```python
from build123d import *

# Parameters (mm, degrees)
SKETCH_1_R          = 4
EXTRUDE_1_DEPTH     = 26
SKETCH_2_R          = 4
EXTRUDE_2_DEPTH     = 36
SKETCH_3_R          = 1.5
CUT_EXTRUDE_1_DEPTH = 37.441734317
CHAMFER_1_SIZE      = 0.2


with BuildPart() as part:
    # ｽｹｯﾁ1 → ﾎﾞｽ - 押し出し1 (new, symmetric)
    with BuildSketch(Plane.XY):
        with Locations(Location((0, 0, 0), (0, 0, 180))):
            Circle(SKETCH_1_R)
    extrude(amount=EXTRUDE_1_DEPTH, both=True)

    # ｽｹｯﾁ2 → ﾎﾞｽ - 押し出し2 (add, symmetric)
    with BuildSketch(Plane.XY):
        with Locations(Location((0, 0, 0), (0, 0, 180))):
            Circle(SKETCH_2_R)
    extrude(amount=EXTRUDE_2_DEPTH, both=True)

    # ｽｹｯﾁ3 → ｶｯﾄ - 押し出し1 (cut, symmetric)
    with BuildSketch(Plane(origin=(0, 0, 0), x_dir=(1, 0, 0), z_dir=(0, 1, 0))):
        with Locations(Location((0, 30, 0), (0, 0, 270))):
            Circle(SKETCH_3_R)
    cut_extrude_1 = extrude(amount=CUT_EXTRUDE_1_DEPTH, both=True, mode=Mode.SUBTRACT)

    # ﾐﾗｰ1: ｶｯﾄ - 押し出し1 across plane
    add(cut_extrude_1.mirror(Plane.XY), mode=Mode.SUBTRACT)

    # 面取り1
    chamfer_1_edges = [part.edges().sort_by_distance(p)[0] for p in [
        (4, 0, -36),
        (4, 0, 36),
    ]]
    chamfer(chamfer_1_edges, length=CHAMFER_1_SIZE)


solid = part.part
```
Verification items for the finished model (mm, model axes). Give positions to 0.01 mm unless a question says otherwise; leave off trailing zeros. Loops run counter-clockwise (first coordinate to the right, second up) from the corner with the lowest first, then second, coordinate; pieces in that order, holes last. Notation, with made-up numbers: M 73,36 L 117,36 A15 ccw 117,64 Z; hole C 37.5,64 d4. An arc over 180 degrees is marked long. One line per question, with ' | ' between items.
Item 1: Section check A-A, the plane y = 0. Record the cut outline in (x, z), plus the area to 3 significant figures.
Completed:
outline: M -4,-35.8 L -3.8,-36 L 3.8,-36 L 4,-35.8 L 4,35.8 L 3.8,36 L -3.8,36 L -4,35.8 Z; hole C 0,-30 d3; hole C 0,30 d3 | area: 562 mm^2
Item 2: Draft check along X on faces 1 (the face through (0.867, 3.905, 0.501)), 2 (the face through (0, 0, -36)), 3 (the face through (0.07, 0.06, -31.5)). Enter one of: +X half, -X half, draft (parallel to the pull), parting line (faces both ways), or undercut.
Completed:
face 1: parting line | face 2: draft | face 3: undercut
Item 3: Section check C-C, the plane z = 30. Record the cut outline in (x, y).
Completed:
outline: M -1.5,-3.71 L -1.5,3.71 A4 ccw Z; M 1.5,-3.71 A4 ccw 1.5,3.71 Z
Item 4: Depth check by flat-ended pin: P1, Ø1, axis at x = 1, z = 9, coming from the +Y side; P2, Ø3, axis at y = 2.5, z = 3.5, coming from the -X side. Enter the tip coordinate at first touch or a pass-through.
Completed:
P1: stops at y = 3.97 | P2: stops at x = -3.87
Item 5: Thickness scan on line 1 (Z direction, x = 0, y = -2.75); line 2 (Z direction, x = 0.5, y = 3.5); line 3 (X direction, y = -1.25, z = 30). Record the ranges inside material, lowest first. Write a range as [from, to].
Completed:
line 1: z = [-36, -31.5], [-28.5, 28.5], [31.5, 36] | line 2: z = [-36, -31.41], [-28.59, 28.59], [31.41, 36] | line 3: x = [-3.8, -1.5], [1.5, 3.8]
Item 6: Section check B-B, the plane z = 22. Record the cut outline in (x, y), plus the area to 3 significant figures.
Completed:
outline: C 0,0 d8 | area: 50.3 mm^2
